Verification items for the finished model (mm, model axes). Face numbers are marked on the shaded views. A direction names the side the tool comes from. Give positions to 0.01 mm unless a question says otherwise; leave off trailing zeros. Order: outer loops, then holes, each group sorted by start corner. A loop starts at its lowest first (then second) coordinate and runs counter-clockwise, first axis right, second up. Notation, with made-up numbers: (-33.75, 6.5) -> (-13.75, 6.5) arc R28 cw to (-13.75, 26.5) -> close; hole circle Ø7 at (13.25, 59). An arc over 180 degrees is marked (long way). Return JSON: item names as keys, results as strings. Group by question number.
(1) Thickness scan on line 1 along Y through (x, z) = (0, 1.25); line 2 along Y through (x, z) = (-13.75, 4.9); line 3 along Y through (x, z) = (13.75, 3.55). Record the ranges inside material, lowest first.
(2) Cross-section at A-A on z = -3.5. Enter the section's corners in (x, y).
(3) Tool access check on the marked faces 1 and 2. Record the directions out of +Z, -Z, +X, -X, +Y, -Y that give a thin tool (end or side, any length) a straight path to the whole face; none if there is none.
(4) Depth check by flat-ended pin: pin 1 Ø1.2 at (y, z) = (-23.5, 1.5) entering from +X; pin 2 Ø0.7 at (y, z) = (-0.5, 1.5) entering from +X; pin 3 Ø6 at (y, z) = (15, 2) entering from -X. Enter the tip coordinate at first touch or a pass-through.
from build123d import *

# Parameters (mm, degrees)
SCHIZZO1_R                   = 30
SCHIZZO1_R_2                 = 21
ESTRUSIONE_ESTRUSIONE1_DEPTH = 4
SCHIZZO2_R                   = 3.05
SCHIZZO3_R                   = 30
SCHIZZO3_R_2                 = 25
ESTRUSIONE_ESTRUSIONE2_DEPTH = 2
TAGLIO_ESTRUSIONE1_START     = -1
SCHIZZO4_R                   = 1.5
TAGLIO_ESTRUSIONE1_DEPTH     = 8
TAGLIO_ESTRUSIONE2_DEPTH     = 2.4
RIPETIZIONECIRCOLARE1_COUNT  = 6
ESTRUSIONE_ESTRUSIONE3_DEPTH = 5


with BuildPart() as part:
    # Schizzo1 → Estrusione-Estrusione1 (new body)
    with BuildSketch(Plane.XY):
        Circle(SCHIZZO1_R)
        Circle(SCHIZZO1_R_2, mode=Mode.SUBTRACT)
    extrude(amount=ESTRUSIONE_ESTRUSIONE1_DEPTH)

    # Schizzo2 → Taglia-Rivoluzione1 (revolve, cut)
    with BuildSketch(Plane(origin=(0, 0, 0), x_dir=(0, 0, -1), z_dir=(1, 0, 0))):
        with Locations((-5.5, 20)):
            Circle(SCHIZZO2_R)
    revolve(axis=Axis((0, 0, 4), (0, 0, -1)), mode=Mode.SUBTRACT)

    # Schizzo3 → Estrusione-Estrusione2 (add)
    with BuildSketch(Plane.XY.offset(4)):
        Circle(SCHIZZO3_R)
        Circle(SCHIZZO3_R_2, mode=Mode.SUBTRACT)
    extrude(amount=ESTRUSIONE_ESTRUSIONE2_DEPTH)

    # Schizzo4 → Taglio-Estrusione1 (cut)
    with BuildSketch(Plane.XY.offset(TAGLIO_ESTRUSIONE1_START)):
        with Locations((-27.5, 0)):
            Circle(SCHIZZO4_R)
    taglio_estrusione1 = extrude(amount=TAGLIO_ESTRUSIONE1_DEPTH, mode=Mode.SUBTRACT)

    # Schizzo5 → Taglio-Estrusione2 (cut)
    with BuildSketch(Plane(origin=(0, 0, 0), x_dir=(-1, 0, 0), z_dir=(0, 0, -1))):
        Polygon((30.25, 1.58771324), (27.5, 3.175426481), (24.75, 1.58771324), (24.75, -1.58771324), (27.5, -3.175426481), (30.25, -1.58771324), align=None)
    taglio_estrusione2 = extrude(amount=-TAGLIO_ESTRUSIONE2_DEPTH, mode=Mode.SUBTRACT)

    # RipetizioneCircolare1: Taglio-Estrusione1, Taglio-Estrusione2 ×6 about axis
    ripetizionecircolare1_axis = Axis((0, 0, 0), (0, 0, 1))
    for i in range(1, RIPETIZIONECIRCOLARE1_COUNT):
        add(taglio_estrusione1.rotate(ripetizionecircolare1_axis, i * 360 / RIPETIZIONECIRCOLARE1_COUNT), mode=Mode.SUBTRACT)
        add(taglio_estrusione2.rotate(ripetizionecircolare1_axis, i * 360 / RIPETIZIONECIRCOLARE1_COUNT), mode=Mode.SUBTRACT)

    # Schizzo6 → Estrusione-Estrusione3 (add)
    with BuildSketch(Plane(origin=(0, 0, 0), x_dir=(-1, 0, 0), z_dir=(0, 0, -1))):
        with BuildLine():
            Line((20.760752105, 3.160881527), (29.658217293, 4.515545038))
            ThreePointArc((29.658217293, 4.515545038), (29.491115616, 5.50219045), (29.291200414, 6.482713806))
            Line((29.291200414, 6.482713806), (20.365348226, 5.123728295))
            ThreePointArc((20.365348226, 5.123728295), (20.586457295, 4.147020139), (20.760752105, 3.160881527))
        make_face()
    extrude(amount=ESTRUSIONE_ESTRUSIONE3_DEPTH)


solid = part.part
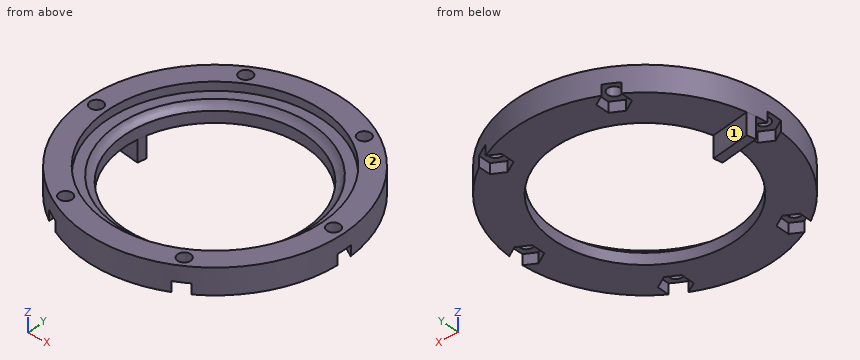
Verdict:
{
 "1": {"line 1": "-30 to -21, 21 to 30", "line 2": "-26.66 to -25.32, -22.32 to -20.88, 20.88 to 22.32, 25.32 to 26.66", "line 3": "-26.66 to -25.32, -22.32 to -17.61, 17.61 to 22.32, 25.32 to 26.66"},
 "2": {"outline": "(-29.66, 4.52) -> (-20.76, 3.16) arc R21 cw to (-20.37, 5.12) -> (-29.29, 6.48) arc R30 ccw to start"},
 "3": {"face 1": "-Z, +X, +Y", "face 2": "+Z, +X, -X, +Y, -Y"},
 "4": {"pin 1": "x = 19.38", "pin 2": "x = 24.75", "pin 3": "x = -27.5"}
}
